```python
from build123d import *

# Parameters (mm, degrees)
F1_DEPTH = 300
F2_T     = -3


with BuildPart() as f1:
    # F0 (on Top) → F1 (new body)
    with BuildSketch(Plane.XY):
        Polygon((0, 650), (0, 0), (655.664250573, 0), (1395.664250573, 376), (1740, 376), (1740, 1026), (1240, 1026), (500, 650), align=None)
    extrude(amount=F1_DEPTH)

    # F2
    f2_openings = [f1.faces().sort_by_distance(p)[0] for p in [
        (0, 325, 150),
        (1740, 701, 150),
    ]]
    offset(amount=F2_T, openings=f2_openings, kind=Kind.INTERSECTION)


solid = f1.part
```
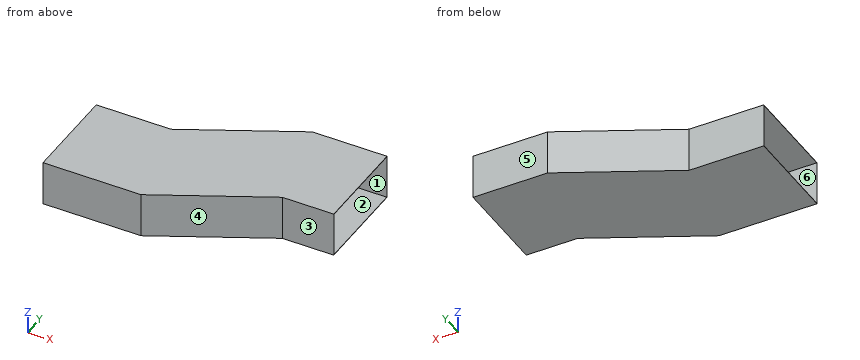
Verification items for the finished model (mm, model axes). Face numbers are marked on the shaded views. A direction names the side the tool comes from. Give positions to 0.01 mm unless a question says otherwise; leave off trailing zeros. Loops run counter-clockwise (first coordinate to the right, second up) from the corner with the lowest first, then second, coordinate; pieces in that order, holes last. Notation, with made-up numbers: M 26,32.25 L 82,32.25 A11 ccw 82,36.25 Z; hole C 58,17 d11. An arc over 180 degrees is marked long. Return JSON: item names as keys, results as strings.
1) Mould release check, pull along Y, two halves, no side actions. Record for the marked faces 4, 5 and 6: released by +Y, released by -Y, zero draft, split by the parting line, or undercut.
Findings:
{"face 4": "released by -Y", "face 5": "released by +Y", "face 6": "undercut"}
2) Section check D-D, the plane y = 776. Enter the section's corners in (x, z), and give its area (3 significant figures).
Findings:
{"outline": "M 747.98,0 L 1740,0 L 1740,3 L 754.6,3 L 754.6,297 L 1740,297 L 1740,300 L 747.98,300 Z", "area": "7,900 mm2"}
3) Section check B-B, the plane y = 414. Enter the section's corners in (x, z), and give its area (3 significant figures).
Findings:
{"outline": "M 0,0 L 1740,0 L 1740,3 L 0,3 Z; M 0,297 L 1740,297 L 1740,300 L 0,300 Z", "area": "10,400 mm2"}
4) Section check C-C, the plane x = 1345. Enter the section's corners in (y, z).
Findings:
{"outline": "M 350.26,0 L 1026,0 L 1026,300 L 350.26,300 Z; hole M 353.62,3 L 1023,3 L 1023,297 L 353.62,297 Z"}
5) Tool access check on the marked faces 1, 2 and 3. Record the directions out of +Z, -Z, +X, -X, +Y, -Y that give a thin tool (end or side, any length) a straight path to the whole face; none if there is none.
Findings:
{"face 1": "+X", "face 2": "none", "face 3": "+Z, -Z, +X, -Y"}
6) Section check A-A, the plane z = 26.5. Enter the section's corners in (x, y), and give its area (3 significant figures).
Findings:
{"outline": "M 0,0 L 655.66,0 L 1395.66,376 L 1740,376 L 1740,379 L 1394.95,379 L 654.95,3 L 0,3 Z; M 0,647 L 500.72,647 L 1240.72,1023 L 1740,1023 L 1740,1026 L 1240,1026 L 500,650 L 0,650 Z", "area": "11,000 mm2"}
7) Material ranges on L1, parallel to Z at x = 1214.5, y = 349; L2, parallel to Y at x = 347.5, z = 21.5; L3, parallel to Y at x = 700, z = 119, recorded low to high. Write a range as [from, to].
Findings:
{"L1": "z = [0, 3], [297, 300]", "L2": "y = [0, 3], [647, 650]", "L3": "y = [22.53, 25.89], [748.26, 751.62]"}
8) Gauge pin test, flat ends, axial feed: P1, Ø8, axis at x = 1071, z = 263.5, coming from the +Y side; P2, Ø5, axis at x = 1563.5, z = 208.5, coming from the -Y side; P3, Ø6, axis at y = 366.5, z = 129.5, coming from the +X side. Record the tip position at first contact, or that the pin passes through.
Findings:
{"P1": "stops at y = 942.16", "P2": "stops at y = 376", "P3": "stops at x = 1382.87"}
